Source: CAD feature listing. Evaluate the final solid. Frame: model axes, mm. A direction names the side the tool comes from. Round coordinates to 2 decimals unless told otherwise and drop trailing zeros. Loops run counter-clockwise (first coordinate to the right, second up) from the corner with the lowest first, then second, coordinate; pieces in that order, holes last.
Item 1: Section query B-B on z = -206. Return loops of the section in (x, y).
Item 2: First-contact query: P1, Ø24, axis at x = 0, y = -74.87, coming from the +Z side; P2, Ø7.5, axis at y = -255.87, z = 5.5, coming from the -X side; P3, Ø3, axis at y = -220, z = -220.5, coming from the +X side; P4, Ø5, axis at y = -258, z = -3, coming from the -X side. Flat tips, straight axial feed; report the tip coordinate or a pass-through.
Item 3: Section query C-C on y = -244. Return loops of the section in (x, z).
Item 4: Section query D-D on x = 0. Return loops of the section in (y, z), then the cut area to 3 significant figures.
Item 5: Access query for faces 1 (the cylindrical face through (-16.3, -262.09, 5.77)), 2 (the flat face through (16.4, -147.9, 75.22)), 3 (the flat face through (-14.613, -181, -96)). Directions: +Z, -Z, +X, -X, +Y, -Y. A direction counts if a zero-diameter tool reaches every point of the face in a straight line with its end or side. Return the directions, or none.
Item 6: Pull-direction query (X, two-part tool) for faces 4 (the flat face through (18.811, -181, -92)), 5 (the cylindrical face through (-16.3, -194.56, 13.35)), 6 (the cylindrical face through (-7.778, -196.778, 104.363)); classes: released by +X, released by -X, zero draft, split by the parting line, or undercut.
Item 7: Section query A-A on y = -150. Return loops of the section in (x, z).
Item 8: Ray query, L1, parallel to X at y = -181, z = -124; L2, parallel to Z at x = 2, y = -269.5; L3, parallel to Y at x = -18, z = -152. Return the intervals inside material, ascending.
```python
from build123d import *

# Parameters (mm, degrees)
F1_DEPTH  = 300
F3_DEPTH  = 300
F4_R      = 6.225
F5_DEPTH  = 200
F6_R      = 7.4994450041
F6_R_2    = 7.7853905485
F7_DEPTH  = 106.4144483809
F9_DEPTH  = 1000
F10_R     = 60.4522878615
F11_DEPTH = 500


with BuildPart() as f1:
    # F0 (on Front) → F1 (new body)
    with BuildSketch(Plane.XZ):
        with BuildLine():
            Line((-18.0362154643, 86.4134483809), (18.8106045383, 86.4134483809))
            Line((18.8106045383, 86.4134483809), (18.8106045383, 78.6302636906))
            ThreePointArc((18.8106045383, 78.6302636906), (19.9890847523, 82.4428187096), (20.387194537, 86.4134483809))
            ThreePointArc((20.387194537, 86.4134483809), (-3.5834351343, 106.0153385962), (-18.0362154643, 78.6302636906))
            Line((-18.0362154643, 78.6302636906), (-18.0362154643, 86.4134483809))
        make_face()
        with BuildLine():
            Line((18.8106045383, 78.6302636906), (18.8106045383, 86.4134483809))
            Line((18.8106045383, 86.4134483809), (-18.0362154643, 86.4134483809))
            Line((-18.0362154643, 86.4134483809), (-18.0362154643, 78.6302636906))
            ThreePointArc((-18.0362154643, 78.6302636906), (0.387194537, 66.4134483809), (18.8106045383, 78.6302636906))
        make_face()
        with BuildLine():
            Line((18.8106045383, -257.5025590471), (18.8106045383, 78.6302636906))
            ThreePointArc((18.8106045383, 78.6302636906), (0.387194537, 66.4134483809), (-18.0362154643, 78.6302636906))
            Line((-18.0362154643, 78.6302636906), (-18.0362154643, -257.5025590471))
            Line((-18.0362154643, -257.5025590471), (18.8106045383, -257.5025590471))
        make_face()
    extrude(amount=F1_DEPTH)

    # F2 (on face) → F3 (cut)
    with BuildSketch(Plane(origin=(0, 0, 0), x_dir=(-1, 0, 0), z_dir=(0, 1, 0))):
        with BuildLine():
            Line((175.8913316219, 44.6973187515), (175.9091161187, 44.6973187515))
            ThreePointArc((175.9091161187, 44.6973187515), (159.7223112701, 60.9808530469), (143.5343522574, 44.6984661409))
            Line((143.5343522574, 44.6984661409), (143.5521367467, 44.6984661409))
            ThreePointArc((143.5521367467, 44.6984661409), (159.6743751329, 60.9629995089), (175.8916158384, 44.7931905997))
            ThreePointArc((175.8916158384, 44.7931905997), (175.8915447841, 44.7452544649), (175.8913316219, 44.6973187515))
        make_face()
        with BuildLine():
            ThreePointArc((174.2740117009, 37.7436316879), (175.4712371526, 41.1301009041), (175.8913316219, 44.6973187515))
            ThreePointArc((175.8913316219, 44.6973187515), (175.8915447841, 44.7452544649), (175.8916158384, 44.7931905997))
            ThreePointArc((175.8916158384, 44.7931905997), (159.6743751329, 60.9629995089), (143.5521367467, 44.6984661409))
            ThreePointArc((143.5521367467, 44.6984661409), (156.1515321138, 29.0223758967), (174.2740117009, 37.7436316879))
        make_face()
        with BuildLine():
            ThreePointArc((14.612805463, 76.6096711506), (16.7870431212, 81.2988018789), (17.5324608163, 86.4134483809))
            ThreePointArc((17.5324608163, 86.4134483809), (-5.501841039, 103.5876860391), (-15.387194537, 76.6096711506))
            Line((-15.387194537, 76.6096711506), (-15.387194537, 86.4134483809))
            Line((-15.387194537, 86.4134483809), (-0.387194537, 86.4134483809))
            Line((-0.387194537, 86.4134483809), (14.612805463, 86.4134483809))
            Line((14.612805463, 86.4134483809), (14.612805463, 76.6096711506))
        make_face()
        with BuildLine():
            Line((-15.387194537, 86.4134483809), (-15.387194537, 76.6096711506))
            ThreePointArc((-15.387194537, 76.6096711506), (-8.9146132219, 70.6528272461), (-0.387194537, 68.4937930276))
            Line((-0.387194537, 68.4937930276), (-0.387194537, 86.4134483809))
            Line((-0.387194537, 86.4134483809), (-15.387194537, 86.4134483809))
        make_face()
        with BuildLine():
            ThreePointArc((-0.387194537, 68.4937930276), (-8.9146132219, 70.6528272461), (-15.387194537, 76.6096711506))
            Line((-15.387194537, 76.6096711506), (-15.387194537, -287.4657809734))
            Line((-15.387194537, -287.4657809734), (-0.387194537, -287.4657809734))
            Line((-0.387194537, -287.4657809734), (-0.387194537, 68.4937930276))
        make_face()
        with BuildLine():
            Line((14.612805463, -287.4657809734), (14.612805463, 76.6096711506))
            ThreePointArc((14.612805463, 76.6096711506), (8.1402241479, 70.6528272461), (-0.387194537, 68.4937930276))
            Line((-0.387194537, 68.4937930276), (-0.387194537, -287.4657809734))
            Line((-0.387194537, -287.4657809734), (14.612805463, -287.4657809734))
        make_face()
        with BuildLine():
            ThreePointArc((-0.387194537, 68.4937930276), (8.1402241479, 70.6528272461), (14.612805463, 76.6096711506))
            Line((14.612805463, 76.6096711506), (14.612805463, 86.4134483809))
            Line((14.612805463, 86.4134483809), (-0.387194537, 86.4134483809))
            Line((-0.387194537, 86.4134483809), (-0.387194537, 68.4937930276))
        make_face()
    extrude(amount=-F3_DEPTH, mode=Mode.SUBTRACT)

    # F4 (on face) → F5 (cut)
    with BuildSketch(Plane.YZ.offset(18.8106045383)):
        with Locations((-286.6114377975, 5.4957243272)):
            Circle(F4_R)
        with Locations((-255.8714377975, 5.4957243272)):
            Circle(F4_R)
        with Locations((-255.8714377975, -218.297693353)):
            Circle(F4_R)
        with Locations((-286.6114377975, -218.297693353)):
            Circle(F4_R)
    extrude(amount=-F5_DEPTH, mode=Mode.SUBTRACT)

    # F6 (on Top) → F7 (cut, through all)
    with BuildSketch(Plane.XY):
        with Locations((0, -74.8674422503)):
            Circle(F6_R)
        with Locations((0, -197.1199959517)):
            Circle(F6_R_2)
    extrude(amount=F7_DEPTH, mode=Mode.SUBTRACT)

    # F8 (on Front) → F9 (cut)
    with BuildSketch(Plane.XZ):
        Polygon((15.4558392242, 69.8942989111), (17.4741577357, 81.283390522), (-16.6930966079, 81.283390522), (-14.6026955917, 69.8942989111), align=None)
    extrude(amount=F9_DEPTH, mode=Mode.SUBTRACT)

    # F10 (on face) → F11 (cut)
    with BuildSketch(Plane.YZ.offset(18.8106045383)):
        Polygon((0, 28.7725478411), (-164.6585613489, -257.5025590471), (0, -257.5025590471), align=None)
        with Locations((-150, -27.5025590471)):
            Circle(F10_R)
    extrude(amount=-F11_DEPTH, mode=Mode.SUBTRACT)


solid = f1.part
```
Data:
1. outline: (-18.04, -300) - (-14.61, -300) - (-14.61, -135.04) - (-18.04, -135.04) - close; (15.39, -300) - (18.81, -300) - (18.81, -135.04) - (15.39, -135.04) - close
2. P1: stops at z = 106.41
2. P2: passes through
2. P3: stops at x = 18.81
2. P4: stops at x = -18.04
3. outline: (-18.04, -257.5) - (-14.61, -257.5) - (-14.61, 69.95) - (-16.57, 80.63) arc R17.92 cw (long way) to (17.37, 80.69) - (15.46, 69.89) - (15.39, 69.89) - (15.39, -257.5) - (18.81, -257.5) - (18.81, 78.63) arc R20 ccw (long way) to (-18.04, 78.63) - close
4. outline: (-300, 104.33) - (-204.91, 104.33) - (-204.91, 106.41) - (-300, 106.41) - close; (-189.33, 104.33) - (-82.37, 104.33) - (-82.37, 106.41) - (-189.33, 106.41) - close; (-67.37, 104.33) - (0, 104.33) - (0, 106.41) - (-67.37, 106.41) - close
4. area: 561 mm2
5. face 1: +X, -X
5. face 2: +Y, -Y
5. face 3: -Z, +Y, -Y
6. face 4: released by +X
6. face 5: zero draft
6. face 6: undercut
7. outline: (-18.04, -232.02) - (-14.61, -232.02) - (-14.61, -87.95) - (-18.04, -87.95) - close; (-18.04, 32.95) - (-14.61, 32.95) - (-14.61, 69.95) - (-16.57, 80.63) arc R17.92 cw (long way) to (17.37, 80.69) - (15.46, 69.89) - (15.39, 69.89) - (15.39, 32.95) - (18.81, 32.95) - (18.81, 78.63) arc R20 ccw (long way) to (-18.04, 78.63) - close; (15.39, -232.02) - (18.81, -232.02) - (18.81, -87.95) - (15.39, -87.95) - close
8. L1: x = -18.04 to -14.61, 15.39 to 18.81
8. L2: z = 104.26 to 106.35
8. L3: y = -300 to -103.98
